from build123d import *

# Parameters (mm, degrees)
F1_DEPTH    = 10
F2_SIZE     = 2.5
F3_T1_DEPTH = 13.9641748973


# Not quite as in the source:
# - a fillet or chamfer that OpenCascade refuses, or shapes differently, is made with other operations: its cross-section is extruded or revolved along the edge and cut away or added


with BuildPart() as f1:
    # F0 (on Front) → F1 (new body)
    with BuildSketch(Plane.XZ):
        with BuildLine():
            Line((4, 36.2801598673), (4, 37.286056375))
            ThreePointArc((4, 37.286056375), (0, 37.5), (-4, 37.286056375))
            Line((-4, 37.286056375), (-4, 36.2801598673))
            ThreePointArc((-4, 36.2801598673), (0, 36.5), (4, 36.2801598673))
        make_face()
    extrude(amount=F1_DEPTH)

    # F2
    f2_edges = [f1.edges().sort_by_distance(p)[0] for p in [
        (-4, -10, 36.783108),
        (-4, 0, 36.783108),
        (4, 0, 36.783108),
        (4, -10, 36.783108),
    ]]
    chamfer(f2_edges, length=F2_SIZE)

    # F3: chamfer of 2.5 on 4 edges, made by hand

    # F3_s2 → F3_t1 (cut)
    with BuildSketch(Plane.XY.offset(29.9874890754)):
        Polygon((-3.267766953, -8.232233047), (1, -10), (-1.5, -10), align=None)
        Polygon((-1, -10), (3.267766953, -8.232233047), (1.5, -10), align=None)
        Polygon((-3.267766953, -1.767766953), (1, 0), (-1.5, 0), align=None)
        Polygon((-1, 0), (3.267766953, -1.767766953), (1.5, 0), align=None)
    extrude(amount=F3_T1_DEPTH, mode=Mode.SUBTRACT)


solid = f1.part
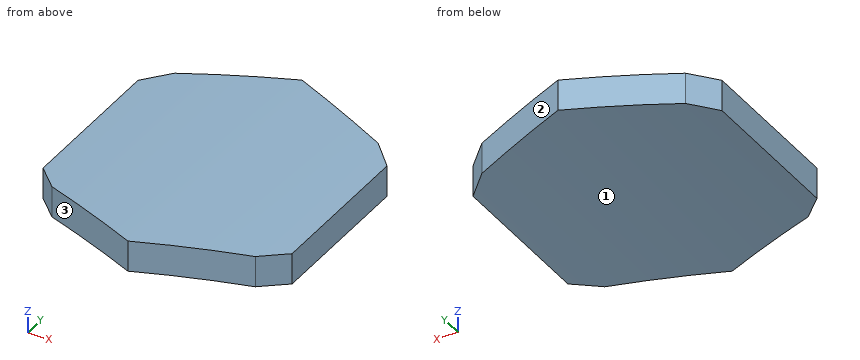
The model under review builds one solid part; all positions refer to its coordinate system, in mm. Face numbers are marked on the shaded views. Round coordinates to 2 decimals unless told otherwise and drop trailing zeros. Loops run counter-clockwise (first coordinate to the right, second up) from the corner with the lowest first, then second, coordinate; pieces in that order, holes last. Notation, with made-up numbers: (66, 78.25) -> (118, 78.25) arc R15 cw to (118, 84.25) -> close; hole circle Ø8 at (-14.5, 72.5). An arc over 180 degrees is marked (long way). Return JSON: item names as keys, results as strings.
(1) Add section A-A on z = 37.1. Write out the cut boundary in (x, y), plus the area to 3 significant figures.
Solved:
{"outline": "(-4, -7.5) -> (-3.27, -8.23) -> (0, -9.59) -> (3.27, -8.23) -> (4, -7.5) -> (4, -2.5) -> (3.27, -1.77) -> (0, -0.41) -> (-3.27, -1.77) -> (-4, -2.5) -> close", "area": "59.5 mm2"}
(2) The part is to be moulded in two halves that separate along X. For the marked faces 1, 2 and 3, say which applies: released by +X, released by -X, zero draft, split by the parting line, or undercut.
Solved:
{"face 1": "undercut", "face 2": "released by +X", "face 3": "released by -X"}
(3) For line 1 (Z direction, x = 3.25, y = -3.75); line 2 (Y direction, x = 3.25, z = 36.55); line 3 (Z direction, x = 1, y = -1), list the stretches that pass through material, from the lowest coordinate up.
Solved:
{"line 1": "36.36 to 37.36", "line 2": "-8.24 to -1.76", "line 3": "36.49 to 37.49"}
(4) For pin 1 (2 mm diameter, centred on x = 1.5, y = -8, fed in from -Z), flat-tipped, find the tip position at first contact; note if it passes through.
Solved:
{"pin 1": "z = 36.41"}
(5) Add section C-C on x = 1.5. Write out the cut boundary in (y, z).
Solved:
{"outline": "(-8.96, 36.47) -> (-1.04, 36.47) -> (-1.04, 37.47) -> (-8.96, 37.47) -> close"}
(6) Add section B-B on y = -4.25. Write out the cut boundary in (x, z), plus the area to 3 significant figures.
Solved:
{"outline": "(-4, 36.28) arc R36.5 cw to (4, 36.28) -> (4, 37.29) arc R37.5 ccw to (-4, 37.29) -> close", "area": "8.02 mm2"}
